The model under review builds one solid part; all positions refer to its coordinate system, in mm. A direction names the side the tool comes from. Round coordinates to 2 decimals unless told otherwise and drop trailing zeros. Loops run counter-clockwise (first coordinate to the right, second up) from the corner with the lowest first, then second, coordinate; pieces in that order, holes last. Notation, with made-up numbers: M -4.75,80.25 L 22.25,80.25 A9 ccw 22.25,91.25 Z; hole C -1,17 d4. An arc over 180 degrees is marked long. Return JSON: item names as keys, results as strings. Group by question number.
Q1. Consider section A-A (y = -2). State the section outline as (x, z) points, and give its area (3 significant figures).
Q2. Clearance check with a flat-ended pin moving along its axis: pin 1 Ø2.5 at (x, y) = (29, -6) entering from -Z. State where the tip first meets the part, or that it passes through.
Q3. For faces 4 (the face through (151, 0, -9)), 5 (the face through (151, 10, 0)), list the 3-axis set-ups (+Z, -Z, +X, -X, +Y, -Y) from which the entire face can be reached by the end or side of a thin tool; tool diameter is ignored.
Q4. To check wall thickness, follow line 1 along Y through (x, z) = (87, -6.5); line 2 along X through (y, z) = (-9.2, -5). State the ranges of each line that lie inside material, in increasing order.
Q5. Draft analysis for pull direction Z (two halves, no side actions). For faces 1 (the face through (151, 0, 9)), 2 (the face through (151, -10, 0)), 3 (the face through (151, 0, -10)), state which applies: pulls with the +Z half, pulls with the -Z half, needs draft (parallel to the pull), parting line crosses it, or undercut.
Q6. Consider section C-C (x = 112.5). State the section outline as (y, z) points.
from build123d import *

# Parameters (mm, degrees)
SKETCH_11_W         = 20
SKETCH_11_H         = 20
SKETCH_11_W_2       = 18
SKETCH_11_H_2       = 18
F_20X20X1_1_DEPTH   = 305.54
SKETCH_16_R         = 1.5
CUT_EXTRUDE_3_DEPTH = 307.357130813
SKETCH_18_R         = 1.5
CUT_EXTRUDE_5_DEPTH = 307.357130813
SKETCH_14_R         = 1.5
CUT_EXTRUDE_6_DEPTH = 20
SKETCH_17_R         = 1.5
CUT_EXTRUDE_7_DEPTH = 20
SKETCH_15_R         = 1.5
CUT_EXTRUDE_8_DEPTH = 20


with BuildPart() as part:
    # 草图11 → 铝管 20X20X1(1) (new body)
    with BuildSketch(Plane(origin=(0, 0, 0), x_dir=(0, 0, -1), z_dir=(1, 0, 0))):
        Rectangle(SKETCH_11_W, SKETCH_11_H)
        Rectangle(SKETCH_11_W_2, SKETCH_11_H_2, mode=Mode.SUBTRACT)
    extrude(amount=F_20X20X1_1_DEPTH)

    # 草图16 → 切除-拉伸3 (cut, through all)
    with BuildSketch(Plane(origin=(0, 0, 10), x_dir=(1, 0, 0), z_dir=(0, 0, -1))):
        with Locations(Location((29, -6, 0), (0, 0, 180))):
            Circle(SKETCH_16_R)
        with Locations(Location((29, 6, 0), (0, 0, 180))):
            Circle(SKETCH_16_R)
    extrude(amount=CUT_EXTRUDE_3_DEPTH, mode=Mode.SUBTRACT)

    # 草图18 → 切除-拉伸5 (cut, through all)
    with BuildSketch(Plane(origin=(0, 10, 0), x_dir=(1, 0, 0), z_dir=(0, 1, 0))):
        with Locations(Location((29, 6, 0), (0, 0, 270))):
            Circle(SKETCH_18_R)
        with Locations(Location((29, -6, 0), (0, 0, 270))):
            Circle(SKETCH_18_R)
    extrude(amount=-CUT_EXTRUDE_5_DEPTH, mode=Mode.SUBTRACT)

    # 草图14 → 切除-拉伸6 (cut)
    with BuildSketch(Plane(origin=(0, 10, 0), x_dir=(1, 0, 0), z_dir=(0, 1, 0))):
        with Locations(Location((294.54, 4.5, 0), (0, 0, 270))):
            Circle(SKETCH_14_R)
        with Locations(Location((294.54, -4.5, 0), (0, 0, 270))):
            Circle(SKETCH_14_R)
    extrude(amount=-CUT_EXTRUDE_6_DEPTH, mode=Mode.SUBTRACT)

    # 草图17 → 切除-拉伸7 (cut)
    with BuildSketch(Plane(origin=(0, 0, -10), x_dir=(-1, 0, 0), z_dir=(0, 0, -1))):
        with Locations((-300.54, 6)):
            Circle(SKETCH_17_R)
        with Locations((-300.54, -6)):
            Circle(SKETCH_17_R)
    extrude(amount=-CUT_EXTRUDE_7_DEPTH, mode=Mode.SUBTRACT)

    # 草图15 → 切除-拉伸8 (cut)
    with BuildSketch(Plane(origin=(0, 10, 0), x_dir=(1, 0, 0), z_dir=(0, 1, 0))):
        with Locations(Location((4, 5, 0), (0, 0, 270))):
            Circle(SKETCH_15_R)
        with Locations(Location((4, -5, 0), (0, 0, 270))):
            Circle(SKETCH_15_R)
        with Locations(Location((18, 5, 0), (0, 0, 270))):
            Circle(SKETCH_15_R)
        with Locations(Location((18, -5, 0), (0, 0, 270))):
            Circle(SKETCH_15_R)
    extrude(amount=-CUT_EXTRUDE_8_DEPTH, mode=Mode.SUBTRACT)


solid = part.part
Values:
{
 "1": {"outline": "M 0,-10 L 305.54,-10 L 305.54,-9 L 0,-9 Z; M 0,9 L 305.54,9 L 305.54,10 L 0,10 Z", "area": "611 mm2"},
 "2": {"pin 1": "passes through"},
 "3": {"face 4": "+X, -X", "face 5": "+Z, -Z, +X, -X, +Y"},
 "4": {"line 1": "y = -10 to -9, 9 to 10", "line 2": "x = 0 to 2.5, 5.5 to 16.5, 19.5 to 27.88, 30.12 to 293.13, 295.95 to 305.54"},
 "5": {"face 1": "undercut", "face 2": "needs draft", "face 3": "pulls with the -Z half"},
 "6": {"outline": "M -10,-10 L 10,-10 L 10,10 L -10,10 Z; hole M -9,-9 L 9,-9 L 9,9 L -9,9 Z"}
}
